Check sheet for the modelled part. Datum: model origin and axes. Units: mm. A direction names the side the tool comes from. Round coordinates to 2 decimals unless told otherwise and drop trailing zeros. Write each loop counter-clockwise with the first axis right and the second up, starting at its lowest first coordinate (ties: lowest second). Pieces come first, ordered by that corner, then holes. Notation, with made-up numbers: M 81,25.5 L 125,25.5 A19 ccw 125,61.5 Z; hole C 31,33.5 d9. An arc over 180 degrees is marked long. One line per item, written item: value.
from build123d import *

# Parameters (mm, degrees)
SKETCH1_W           = 80
SKETCH1_H           = 80
BOSS_EXTRUDE1_DEPTH = 4
FILLET3_R           = 3
FILLET2_R           = 3
SKETCH3_R           = 35
BOSS_EXTRUDE3_DEPTH = 17
SKETCH4_W           = 80
SKETCH4_H           = 80
BOSS_EXTRUDE4_DEPTH = 4
FILLET4_R           = 3
SKETCH5_R           = 30
CUT_EXTRUDE1_DEPTH  = 71.455659815
SKETCH6_R           = 5
CUT_EXTRUDE2_DEPTH  = 71.455659815


with BuildPart() as part:
    # Sketch1 → Boss-Extrude1 (new body)
    with BuildSketch(Plane(origin=(0, 0, 0), x_dir=(1, 0, 0), z_dir=(0, 1, 0))):
        Rectangle(SKETCH1_W, SKETCH1_H)
    extrude(amount=BOSS_EXTRUDE1_DEPTH)

    # Fillet3
    fillet3_edges = [part.edges().sort_by_distance(p)[0] for p in [
        (40, 2, 40),
    ]]
    fillet(fillet3_edges, radius=FILLET3_R)

    # Fillet2
    fillet2_edges = [part.edges().sort_by_distance(p)[0] for p in [
        (-40, 2, -40),
        (40, 2, -40),
        (-40, 2, 40),
    ]]
    fillet(fillet2_edges, radius=FILLET2_R)

    # Sketch3 → Boss-Extrude3 (add)
    with BuildSketch(Plane(origin=(0, 4, 0), x_dir=(1, 0, 0), z_dir=(0, 1, 0))):
        with Locations(Location((0, 0, 0), (0, 0, 270))):
            Circle(SKETCH3_R)
    boss_extrude3 = extrude(amount=BOSS_EXTRUDE3_DEPTH)

    # Mirror1: Boss-Extrude3 across plane
    add(boss_extrude3.mirror(Plane.ZX.offset(21)))

    # Sketch4 → Boss-Extrude4 (add)
    with BuildSketch(Plane(origin=(0, 38, 0), x_dir=(1, 0, 0), z_dir=(0, 1, 0))):
        Rectangle(SKETCH4_W, SKETCH4_H)
    extrude(amount=BOSS_EXTRUDE4_DEPTH)

    # Fillet4
    fillet4_edges = [part.edges().sort_by_distance(p)[0] for p in [
        (-40, 40, -40),
        (-40, 40, 40),
        (40, 40, 40),
        (40, 40, -40),
    ]]
    fillet(fillet4_edges, radius=FILLET4_R)

    # Sketch5 → Cut-Extrude1 (cut, through all)
    with BuildSketch(Plane(origin=(0, 42, 0), x_dir=(1, 0, 0), z_dir=(0, 1, 0))):
        with Locations(Location((0, 0, 0), (0, 0, 270))):
            Circle(SKETCH5_R)
    extrude(amount=-CUT_EXTRUDE1_DEPTH, mode=Mode.SUBTRACT)

    # Sketch6 → Cut-Extrude2 (cut, through all)
    with BuildSketch(Plane(origin=(0, 42, 0), x_dir=(1, 0, 0), z_dir=(0, 1, 0))):
        with Locations(Location((30, 30, 0), (0, 0, 270))):
            Circle(SKETCH6_R)
        with Locations(Location((30, -30, 0), (0, 0, 270))):
            Circle(SKETCH6_R)
        with Locations(Location((-30, -30, 0), (0, 0, 270))):
            Circle(SKETCH6_R)
        with Locations(Location((-30, 30, 0), (0, 0, 270))):
            Circle(SKETCH6_R)
    extrude(amount=-CUT_EXTRUDE2_DEPTH, mode=Mode.SUBTRACT)


solid = part.part
Q1. Scan lines: line 1 (X direction, y = 25.5, z = 0); line 2 (X direction, y = 18.5, z = -10.5); line 3 (Z direction, x = -24.5, y = 23) (3 decimals). Record each from-to range of solid material in increasing order. Write a range as [from, to].
Completed:
line 1: [-35, -30], [30, 35]
line 2: [-33.39, -28.1], [28.1, 33.39]
line 3: [-24.995, -17.313], [17.313, 24.995]
Q2. Depth check by flat-ended pin: P1, Ø1.5, axis at x = 21, y = 20, coming from the -Z side; P2, Ø10, axis at y = 20, z = -15, coming from the +X side; P3, Ø5, axis at y = 34.5, z = -4, coming from the +X side. Enter the tip coordinate at first touch or a pass-through.
Completed:
P1: z = -28.55
P2: x = 33.54
P3: x = 34.97
Q3. Sectioned sample at A-A on x = 0. Enter the section's corners in (y, z), and give its area (3 significant figures).
Completed:
outline: M 0,-40 L 4,-40 L 4,-35 L 38,-35 L 38,-40 L 42,-40 L 42,-30 L 0,-30 Z; M 0,30 L 42,30 L 42,40 L 38,40 L 38,35 L 4,35 L 4,40 L 0,40 Z
area: 500 mm^2
Q4. Sectioned sample at B-B on z = 0. Enter the section's corners in (x, y).
Completed:
outline: M -40,0 L -30,0 L -30,42 L -40,42 L -40,38 L -35,38 L -35,4 L -40,4 Z; M 30,0 L 40,0 L 40,4 L 35,4 L 35,38 L 40,38 L 40,42 L 30,42 Z
Q5. Sectioned sample at D-D on y = 27. Enter the section's corners in (x, z).
Completed:
outline: C 0,0 d70; hole C 0,0 d60
Q6. Sectioned sample at C-C on x = 26. State how many separate pieces and enclosed holes the cut face has, and give its area (3 significant figures).
Completed:
separate pieces: 6
enclosed holes: 0
area: 880 mm^2
Q7. Draft check along X on faces 3 (the cylindrical face through (27, 2, -34)), 4 (the cylindrical face through (39.14, 2.03, -39.1)), 5 (the cylindrical face through (-39.14, 40.03, 39.1)). Enter one of: pulls with the +X half, pulls with the -X half, needs draft (parallel to the pull), parting line crosses it, or undercut.
Completed:
face 3: undercut
face 4: pulls with the +X half
face 5: pulls with the -X half
Q8. Access from +Z, -Z, +X, -X, +Y, -Y to the whole of each face (thin tool, end or side, straight path). Record for faces 1 (the cylindrical face through (-30, 40, 25)), 2 (the flat face through (8, 38, 35)).
Completed:
face 1: +Y, -Y
face 2: none
